Geometry: final body of the model. Coordinates: model frame, mm. Face numbers are marked on the shaded views. Give positions to 0.01 mm unless a question says otherwise; leave off trailing zeros. Write each loop counter-clockwise with the first axis right and the second up, starting at its lowest first coordinate (ties: lowest second). Pieces come first, ordered by that corner, then holes.
Q1. Section B-B (y = 22.5). State how many separate pieces and enclosed holes the cut face has, plus the area to 3 significant figures.
Q2. Mould query, pull axis X, two halves, no side actions, for the marked faces 1 and 2. Classes: +X half, -X half, draft (parallel to the pull), parting line (faces both ways), or undercut.
Q3. Pin query (flat end, axial travel): pin 1 Ø1 at (y, z) = (30.5, 6) entering from +X; pin 2 Ø14 at (x, y) = (30, 25.21) entering from -Z; pin 3 Ø1 at (y, z) = (10, 8) entering from +X. Return the tip coordinate at first contact, or that it passes through.
Q4. Section C-C (z = 1.5). Return the cut outline in (x, y), plus the area to 3 significant figures.
Q5. Line query: line 1 (X direction, y = 23.5, z = 7); line 2 (X direction, y = 29, z = 8); line 3 (X direction, y = 44, z = 5.5). Output: solid intervals per line, ascending.
from build123d import *

# Parameters (mm, degrees)
ESBO_O1_W                                = 190
ESBO_O1_H                                = 50
RESSALTO_EXTRUS_O1_DEPTH                 = 10
FILETE1_R                                = 5
BROCA_DE_ROSQUEAR_PARA_TARRAXA_DE_M201_D = 17.5


with BuildPart() as part:
    # Esboço1 → Ressalto-extrusão1 (new body)
    with BuildSketch(Plane.XY):
        with Locations((95, 25)):
            Rectangle(ESBO_O1_W, ESBO_O1_H)
    extrude(amount=RESSALTO_EXTRUS_O1_DEPTH)

    # Filete1
    filete1_edges = [part.edges().sort_by_distance(p)[0] for p in [
        (95, 50, 10),
        (0, 25, 10),
        (95, 0, 10),
        (0, 25, 0),
        (95, 50, 0),
        (190, 25, 0),
        (95, 0, 0),
        (0, 0, 5),
        (0, 50, 5),
        (190, 50, 5),
        (190, 0, 5),
        (190, 25, 10),
    ]]
    fillet(filete1_edges, radius=FILETE1_R - 0.0001)  # a hair under: the kernel refuses the full size

    # Broca de rosquear para tarraxa de M201 (through all)
    with Locations(Plane.XY.offset(10)):
        with Locations((30, 25.206865572), (160, 25.206865572)):
            Hole(BROCA_DE_ROSQUEAR_PARA_TARRAXA_DE_M201_D / 2)


solid = part.part
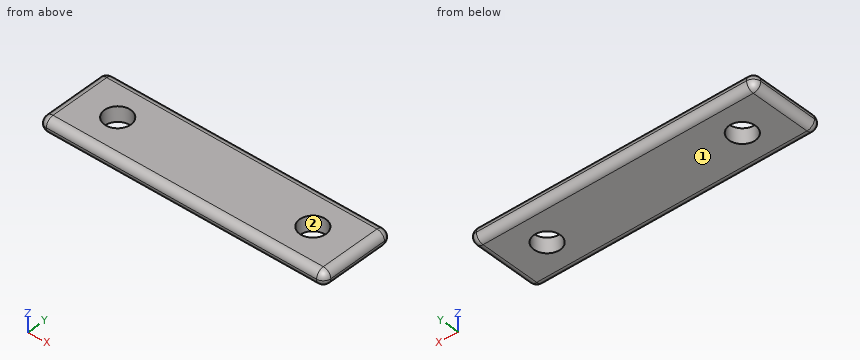
Computed:
1. separate pieces: 3
1. enclosed holes: 0
1. area: 1,550 mm2
2. face 1: draft
2. face 2: undercut
3. pin 1: stops at x = 189.97
3. pin 2: passes through
3. pin 3: stops at x = 189.33
4. outline: (1.43, 5) arc R3.57 ccw to (5, 1.43) - (185, 1.43) arc R3.57 ccw to (188.57, 5) - (188.57, 45) arc R3.57 ccw to (185, 48.57) - (5, 48.57) arc R3.57 ccw to (1.43, 45) - close; hole circle Ø17.5 at (30, 25.21); hole circle Ø17.5 at (160, 25.21)
4. area: 8,330 mm2
5. line 1: x = 0.42 to 21.42, 38.58 to 151.42, 168.58 to 189.58
5. line 2: x = 1 to 22.11, 37.89 to 152.11, 167.89 to 189
5. line 3: x = 0.03 to 189.97
